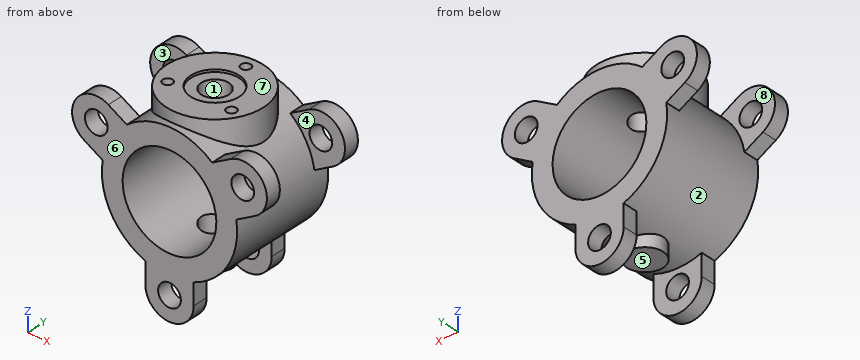
from build123d import *

# Parameters (mm, degrees)
SKETCH1_R                = 140
SKETCH1_R_2              = 97
BOSS_EXTRUDE1_DEPTH      = 112.5
BOSS_EXTRUDE2_REACH      = 353.799
BOSS_EXTRUDE2_END_RADIUS = 140
SKETCH2_R                = 100
BOSS_EXTRUDE3_REACH      = 373.324
BOSS_EXTRUDE3_END_RADIUS = 140
SKETCH3_R                = 37.5
HOLE1_D                  = 20.3
HOLE1_DEPTH              = 30
CIRPATTERN2_COUNT        = 3
HOLE2_D                  = 56.2
HOLE2_DEPTH              = 310
HOLE2_CBORE_D            = 100
HOLE2_CBORE_DEPTH        = 5
BOSS_EXTRUDE6_DEPTH      = 32
CIRPATTERN5_COUNT        = 3
SKETCH16_W               = 23.5
SKETCH16_H               = 32
HOLE3_AT_2_COUNT         = 2
HOLE3_AT_2_PITCH         = 303.108891325
HOLE3_AT_3_COUNT         = 2
HOLE3_AT_3_PITCH         = 303.108891325
MIRROR1_COPY_1_DEPTH     = 32
MIRROR1_COPY_2_DEPTH     = 32
MIRROR1_COPY_3_SKETCH_W  = 23.5
MIRROR1_COPY_3_SKETCH_H  = 32
MIRROR1_COPY_4_SKETCH_W  = 23.5
MIRROR1_COPY_4_SKETCH_H  = 32


with BuildPart() as part:
    # Sketch1 → Boss-Extrude1 (new, symmetric)
    with BuildSketch(Plane(origin=(0, 0, 0), x_dir=(1, 0, 0), z_dir=(0, 1, 0))):
        with Locations(Location((0, 0, 0), (0, 0, 270))):
            Circle(SKETCH1_R)
        with Locations(Location((0, 0, 0), (0, 0, 270))):
            Circle(SKETCH1_R_2, mode=Mode.SUBTRACT)
    extrude(amount=BOSS_EXTRUDE1_DEPTH, both=True)

    # Boss-Extrude2: up to this cylinder (the profile starts outside it)
    boss_extrude2_end = Plane(origin=(0, 0, 0), z_dir=(0, -1, 0)) * Cylinder(BOSS_EXTRUDE2_END_RADIUS, 988.598, mode=Mode.PRIVATE)
    # Sketch2 → Boss-Extrude2 (add, up to the surface)
    with BuildSketch(Plane.XY.offset(162.5), mode=Mode.PRIVATE) as boss_extrude2_sk1:
        Circle(SKETCH2_R)
    boss_extrude2_tool1 = extrude(boss_extrude2_sk1.sketch, amount=-BOSS_EXTRUDE2_REACH, mode=Mode.PRIVATE) - boss_extrude2_end
    add(boss_extrude2_tool1.solids().sort_by_distance((0, 0, 162.5))[0])

    # Boss-Extrude3: up to this cylinder (the profile starts outside it)
    boss_extrude3_end = Plane(origin=(0, 0, 0), z_dir=(0, -1, 0)) * Cylinder(BOSS_EXTRUDE3_END_RADIUS, 1027.648, mode=Mode.PRIVATE)
    # Sketch3 → Boss-Extrude3 (add, up to the surface)
    with BuildSketch(Plane.XY.offset(-162.5), mode=Mode.PRIVATE) as boss_extrude3_sk1:
        with Locations(Location((0, 0, 0), (0, 0, 90))):
            Circle(SKETCH3_R)
    boss_extrude3_tool1 = extrude(boss_extrude3_sk1.sketch, amount=BOSS_EXTRUDE3_REACH, mode=Mode.PRIVATE) - boss_extrude3_end
    add(boss_extrude3_tool1.solids().sort_by_distance((0, 0, -162.5))[0])

    # Hole1
    with Locations(Plane.XY.offset(162.5)):
        with Locations((0, 76.3)):
            hole1 = Hole(HOLE1_D / 2, depth=HOLE1_DEPTH)

    # CirPattern2: Hole1 ×3 about axis
    cirpattern2_axis = Axis((0, 0, 0), (0, 0, 1))
    for i in range(1, CIRPATTERN2_COUNT):
        add(hole1.rotate(cirpattern2_axis, i * 360 / CIRPATTERN2_COUNT), mode=Mode.SUBTRACT)

    # Hole2
    with Locations(Plane.XY.offset(162.5)):
        with Locations((0, 0)):
            CounterBoreHole(HOLE2_D / 2, HOLE2_CBORE_D / 2, HOLE2_CBORE_DEPTH, depth=HOLE2_DEPTH)

    # Sketch10 → Boss-Extrude6 (add)
    with BuildSketch(Plane(origin=(0, 112.5, 0), x_dir=(1, 0, 0), z_dir=(0, 1, 0))):
        with BuildLine():
            Line((50, 130.766968306), (50, 175))
            ThreePointArc((50, 175), (0, 225), (-50, 175))
            Line((-50, 175), (-50, 130.766968306))
            ThreePointArc((-50, 130.766968306), (0, 140), (50, 130.766968306))
        make_face()
    boss_extrude6 = extrude(amount=-BOSS_EXTRUDE6_DEPTH)

    # CirPattern5: Boss-Extrude6 ×3 about axis
    cirpattern5_axis = Axis((0, 0, 0), (0, 1, 0))
    for i in range(1, CIRPATTERN5_COUNT):
        add(boss_extrude6.rotate(cirpattern5_axis, i * 360 / CIRPATTERN5_COUNT))

    # Sketch16 → Hole3 (revolve, cut)
    with BuildSketch(Plane(origin=(0, 112.5, -175), x_dir=(0, 0, 1), z_dir=(1, 0, 0))):
        with Locations((11.75, 16)):
            Rectangle(SKETCH16_W, SKETCH16_H)
    hole3 = revolve(axis=Axis((0, 2.5, -175), (0, 1, 0)), mode=Mode.SUBTRACT)

    # Hole3 at 2: Hole3 ×2
    with Locations(*[Vector(0.500000000000004, 0, 0.8660254037844364) * (i * HOLE3_AT_2_PITCH) for i in range(1, HOLE3_AT_2_COUNT)]):
        add(hole3, mode=Mode.SUBTRACT)

    # Hole3 at 3: Hole3 ×2
    with Locations(*[Vector(-0.49999999999999806, 0, 0.8660254037844397) * (i * HOLE3_AT_3_PITCH) for i in range(1, HOLE3_AT_3_COUNT)]):
        add(hole3, mode=Mode.SUBTRACT)

    # Mirror1: Boss-Extrude6, Hole3 across plane
    add(boss_extrude6.mirror(Plane.ZX))
    add(hole3.mirror(Plane.ZX), mode=Mode.SUBTRACT)

    # Mirror1 copy 1 sketch → Mirror1 copy 1 (add)
    with BuildSketch(Plane(origin=(0, -112.5, 0), x_dir=(-0.4999999999999998, 0, -0.8660254037844387), z_dir=(0, -1, 0))):
        with BuildLine():
            Line((50, -130.766968306), (50, -175))
            ThreePointArc((50, -175), (0, -225), (-50, -175))
            Line((-50, -175), (-50, -130.766968306))
            ThreePointArc((-50, -130.766968306), (0, -140), (50, -130.766968306))
        make_face()
    extrude(amount=-MIRROR1_COPY_1_DEPTH)

    # Mirror1 copy 2 sketch → Mirror1 copy 2 (add)
    with BuildSketch(Plane(origin=(0, -112.5, 0), x_dir=(-0.5000000000000004, 0, 0.8660254037844384), z_dir=(0, -1, 0))):
        with BuildLine():
            Line((50, -130.766968306), (50, -175))
            ThreePointArc((50, -175), (0, -225), (-50, -175))
            Line((-50, -175), (-50, -130.766968306))
            ThreePointArc((-50, -130.766968306), (0, -140), (50, -130.766968306))
        make_face()
    extrude(amount=-MIRROR1_COPY_2_DEPTH)

    # Mirror1 copy 3 sketch → Mirror1 copy 3 (revolve, cut)
    with BuildSketch(Plane(origin=(151.554445662, -112.5, 87.5), x_dir=(0, 0, 1), z_dir=(1, 0, 0))):
        with Locations((11.75, -16)):
            Rectangle(MIRROR1_COPY_3_SKETCH_W, MIRROR1_COPY_3_SKETCH_H)
    revolve(axis=Axis((151.554445662, -2.5, 87.5), (0, 1, 0)), mode=Mode.SUBTRACT)

    # Mirror1 copy 4 sketch → Mirror1 copy 4 (revolve, cut)
    with BuildSketch(Plane(origin=(-151.554445662, -112.5, 87.5), x_dir=(0, 0, 1), z_dir=(1, 0, 0))):
        with Locations((11.75, -16)):
            Rectangle(MIRROR1_COPY_4_SKETCH_W, MIRROR1_COPY_4_SKETCH_H)
    revolve(axis=Axis((-151.554445662, -2.5, 87.5), (0, 1, 0)), mode=Mode.SUBTRACT)


solid = part.part
The listing builds one solid part. Answer for the finished solid, in the listing's coordinates (mm). Face numbers are marked on the shaded views. A direction names the side the tool comes from. Give positions to 0.01 mm unless a question says otherwise; leave off trailing zeros. Write each loop counter-clockwise with the first axis right and the second up, starting at its lowest first coordinate (ties: lowest second). Pieces come first, ordered by that corner, then holes.
Item 1: Section D-D, the plane z = 87.5 is taken. Count the separate pieces of the cut face and the enclosed holes in it, plus the area to 3 significant figures.
Item 2: Which of the six approach directions +Z, -Z, +X, -X, +Y, -Y give full straight-line access (tool end or side, diameter ignored) to the marked faces 1, 2, 3, 4 and 5?
Item 3: Determine the mould class of the marked faces 6, 7 and 8 for opening direction Y: released by +Y, released by -Y, zero draft, split by the parting line, or undercut.
Item 4: Flat-ended cylindrical pins translate along their axes: P1, Ø6, axis at y = 58.5, z = 13, coming from the -X side; P2, Ø9.5, axis at y = -90, z = -146, coming from the +X side; P3, Ø8, axis at x = -20, z = -182.5, coming from the +Y side; P4, Ø12, axis at y = -8.5, z = 7, coming from the -X side. Find the tip coordinate at first contact, or state that the pin passes through.
Item 5: Find the intervals of material crossed by line 1 along Z through (x, y) = (2, -97); line 2 along Z through (x, y) = (-6.5, -88.5); line 3 along X through (y, z) = (-95, 87), in increasing order.
Item 6: Section C-C, the plane x = -43.5 is taken. Write down the section's boundary in (y, z), plus the area to 3 significant figures.
Item 7: Section A-A, the plane z = 0 is taken. Write down the section's boundary in (x, y).
Item 8: Section B-B, the plane y = 0 is taken. Write down the section's boundary in (x, z), plus the area to 3 significant figures.
Completed:
1. separate pieces: 6
1. enclosed holes: 0
1. area: 36,100 mm2
2. face 1: +Z
2. face 2: none
2. face 3: +Z, -X
2. face 4: +Z, +X
2. face 5: -Z, +X, -X
3. face 6: released by -Y
3. face 7: zero draft
3. face 8: undercut
4. P1: stops at x = -139.64
4. P2: stops at x = 50
4. P3: stops at y = 112.5
4. P4: stops at x = -140
5. line 1: z = -224.96 to -198.41, -151.59 to -96.98, 96.98 to 162.5
5. line 2: z = -224.58 to -197.58, -152.42 to -96.78, 96.78 to 162.5
5. line 3: x = -201.55 to -175.05, -128.06 to -42.9, 42.9 to 128.06, 175.05 to 201.55
6. outline: (-112.5, -199.65) - (-80.5, -199.65) - (-80.5, -133.07) - (80.5, -133.07) - (80.5, -199.65) - (112.5, -199.65) - (112.5, -86.7) - (-112.5, -86.7) - close; (-112.5, 86.7) - (112.5, 86.7) - (112.5, 133.07) - (90.04, 133.07) - (90.04, 162.5) - (24.65, 162.5) - (24.65, 157.5) - (-24.65, 157.5) - (-24.65, 162.5) - (-90.04, 162.5) - (-90.04, 133.07) - (-112.5, 133.07) - close
6. area: 30,200 mm2
7. outline: (-140, -112.5) - (-97, -112.5) - (-97, 112.5) - (-140, 112.5) - close; (97, -112.5) - (140, -112.5) - (140, 112.5) - (97, 112.5) - close
8. outline: (-100, 97.98) arc R140 ccw to (-37.5, -134.88) - (-37.5, -162.5) - (37.5, -162.5) - (37.5, -134.88) arc R140 ccw to (100, 97.98) - (100, 162.5) - (50, 162.5) - (50, 157.5) - (28.1, 157.5) - (28.1, 92.84) arc R97 cw to (28.1, -92.84) - (28.1, -147.5) - (-28.1, -147.5) - (-28.1, -92.84) arc R97 cw to (-28.1, 92.84) - (-28.1, 157.5) - (-50, 157.5) - (-50, 162.5) - (-100, 162.5) - close
8. area: 34,000 mm2
